from build123d import *

# Parameters (mm, degrees)
PAD_DEPTH = 10


with BuildPart() as part:
    # Sketch → Pad (new body)
    with BuildSketch(Plane.XY):
        with BuildLine():
            Line((-3, 30), (-3, 0))
            Line((-3, 0), (-1.500009, 0))
            ThreePointArc((-1.500009, 0), (-0.439343, 0.439336), (0, 1.499999))
            Line((0, 1.499999), (0, 25.5))
            ThreePointArc((1.5, 27), (0.43934, 26.56066), (0, 25.5))
            Line((1.5, 27), (7.5, 27))
            ThreePointArc((9, 25.5), (8.56066, 26.56066), (7.5, 27))
            Line((9, 25.5), (9, 9.5))
            ThreePointArc((7.5, 8), (8.56066, 8.43934), (9, 9.5))
            Line((6.5, 8), (7.5, 8))
            ThreePointArc((6.5, 8), (5, 6.5), (6.5, 5))
            Line((6.5, 5), (10.5, 5))
            ThreePointArc((10.5, 5), (11.56066, 5.43934), (12, 6.5))
            Line((12, 6.5), (12, 28.500001))
            ThreePointArc((12, 28.500001), (11.56066, 29.560661), (10.5, 30))
            Line((-3, 30), (10.5, 30))
        make_face()
    extrude(amount=PAD_DEPTH)


solid = part.part
For this review, take the finished solid that the model builds, in its own axes (mm). A direction names the side the tool comes from. Give positions to 0.01 mm unless a question says otherwise; leave off trailing zeros. Loops run counter-clockwise (first coordinate to the right, second up) from the corner with the lowest first, then second, coordinate; pieces in that order, holes last.
Item 1: Tool access review of faces 5 (the cylindrical face through (0.45, 26.57, 4.93)), 6 (the flat face through (8, 5, 5)), 7 (the flat face through (4, 27, 5)): name each direction out of +Z, -Z, +X, -X, +Y, -Y from which nothing blocks a thin tool from reaching the whole face with its end or side.
Item 2: Insertion check: pin 1 (2 mm diameter, centred on x = 8.5, z = 4, fed in from -Y); pin 2 (2 mm diameter, centred on x = 3.5, z = 8, fed in from -Y); pin 3 (3 mm diameter, centred on x = 4.5, z = 6.5, fed in from -Y). Each pin has a flat end and moves straight along its axis. Give the tip position at first contact, or say it passes through.
Item 3: Take a section at D-D, the plane x = 9.75. State the section outline as (y, z) points.
Item 4: Take a section at B-B, the plane y = 15.5. State the section outline as (x, z) points, and give its area (3 significant figures).
Item 5: Take a section at C-C, the plane z = 1.75. State the section outline as (x, y) points.
Item 6: Take a section at A-A, the plane x = 7. State the section outline as (y, z) points, and give its area (3 significant figures).
Item 7: Draft analysis for pull direction Y (two halves, no side actions). For faces 1 (the cylindrical face through (11.57, 29.55, 4.93)), 2 (the cylindrical face through (8.57, 26.55, 4.93)), 3 (the flat face through (0, 13, 5)), 4 (the cylindrical face through (5, 6.5, 4.9)), state which applies: +Y half, -Y half, draft (parallel to the pull), parting line (faces both ways), or undercut.
Item 8: For line 1 along X through (y, z) = (22, 2.5); line 2 along Y through (x, z) = (2, 9.25); line 3 along X through (y, z) = (2.5, 4), list the stretches that pass through material, from the lowest coordinate up.
Calculated:
1. face 5: +Z, -Z, -Y
1. face 6: +Z, -Z, +X, -Y
1. face 7: +Z, -Z
2. pin 1: stops at y = 5
2. pin 2: stops at y = 27
2. pin 3: stops at y = 5.09
3. outline: (5, 0) - (30, 0) - (30, 10) - (5, 10) - close
4. outline: (-3, 0) - (0, 0) - (0, 10) - (-3, 10) - close; (9, 0) - (12, 0) - (12, 10) - (9, 10) - close
4. area: 60.0 mm2
5. outline: (-3, 0) - (-1.5, 0) arc R1.5 ccw to (0, 1.5) - (0, 25.5) arc R1.5 cw to (1.5, 27) - (7.5, 27) arc R1.5 cw to (9, 25.5) - (9, 9.5) arc R1.5 cw to (7.5, 8) - (6.5, 8) arc R1.5 ccw to (6.5, 5) - (10.5, 5) arc R1.5 ccw to (12, 6.5) - (12, 28.5) arc R1.5 ccw to (10.5, 30) - (-3, 30) - close
6. outline: (5, 0) - (8, 0) - (8, 10) - (5, 10) - close; (27, 0) - (30, 0) - (30, 10) - (27, 10) - close
6. area: 60.0 mm2
7. face 1: +Y half
7. face 2: undercut
7. face 3: draft
7. face 4: undercut
8. line 1: x = -3 to 0, 9 to 12
8. line 2: y = 27 to 30
8. line 3: x = -3 to 0
